Geometry: see drawing. Coordinates: mm, zero at the bounding-box minimum. A direction names the side the tool comes from. Give positions to 0.01 mm unless a question says otherwise; leave off trailing zeros. Loops run counter-clockwise (first coordinate to the right, second up) from the corner with the lowest first, then second, coordinate; pieces in that order, holes last. Notation, with made-up numbers: M 18.5,-17 L 55.5,-17 A14 ccw 55.5,2 Z; hole C 22.5,-9.5 d1. An arc over 180 degrees is marked long. Put each result on its own line as item: value.
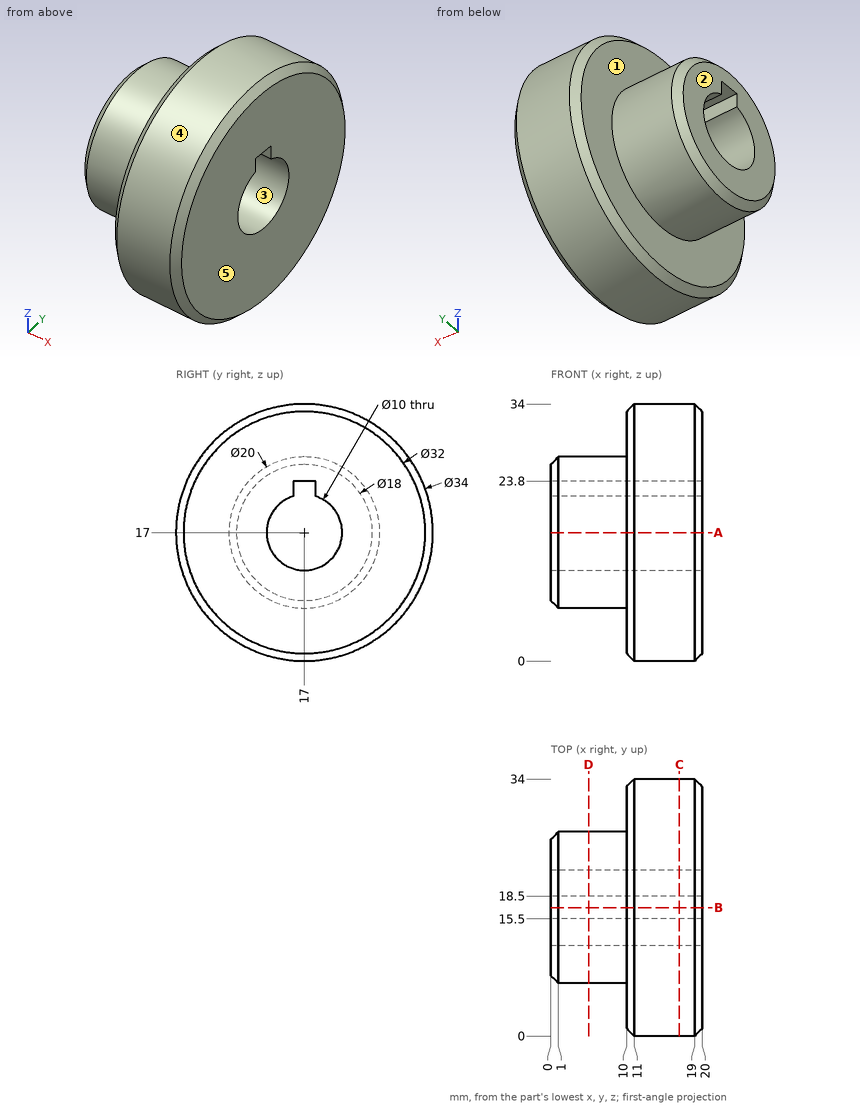
1. Material intervals for line 1 (Y direction, x = 16, z = 17); line 2 (Z direction, x = 4.75, y = 17); line 3 (Z direction, x = 12.5, y = 17), sorted ascending. Write a range as from..to.
Found:
line 1: 0..12, 22..34
line 2: 7..12, 23.8..27
line 3: 0..12, 23.8..34
2. Section query B-B (y = 17). Output: boundary loops of the cut face in (x, z).
Found:
outline: M 0,8 L 1,7 L 10,7 L 10,1 L 11,0 L 19,0 L 20,1 L 20,12 L 0,12 Z; M 0,23.8 L 20,23.8 L 20,33 L 19,34 L 11,34 L 10,33 L 10,27 L 1,27 L 0,26 Z
3. Access query for the marked faces 1 and 2. Directions: +Z, -Z, +X, -X, +Y, -Y. A direction counts if a zero-diameter tool reaches every point of the face in a straight line with its end or side. Return the directions, or none.
Found:
face 1: -X
face 2: +Z, -Z, -X, +Y, -Y
4. Section query D-D (x = 5). Output: boundary loops of the cut face in (y, z), plus the area to 3 significant figures.
Found:
outline: C 17,17 d20; hole M 15.5,21.77 A5 ccw long 18.5,21.77 L 18.5,23.8 L 15.5,23.8 Z
area: 230 mm^2
5. Section query C-C (x = 17). Output: boundary loops of the cut face in (y, z), plus the area to 3 significant figures.
Found:
outline: C 17,17 d34; hole M 15.5,21.77 A5 ccw long 18.5,21.77 L 18.5,23.8 L 15.5,23.8 Z
area: 824 mm^2
6. Section query A-A (z = 17). Output: boundary loops of the cut face in (x, y), plus the area to 3 significant figures.
Found:
outline: M 0,8 L 1,7 L 10,7 L 10,1 L 11,0 L 19,0 L 20,1 L 20,12 L 0,12 Z; M 0,22 L 20,22 L 20,33 L 19,34 L 11,34 L 10,33 L 10,27 L 1,27 L 0,26 Z
area: 337 mm^2
7. Draft query along Z for the marked faces 3, 4 and 5. Return one class per face: pulls with the +Z half, pulls with the -Z half, needs draft (parallel to the pull), parting line crosses it, or undercut.
Found:
face 3: undercut
face 4: parting line crosses it
face 5: needs draft
8. Contact query for flat-ended pins moving along their axis: P1, Ø6, axis at y = 17, z = 17, coming from the +X side; P2, Ø8, axis at x = 11.5, z = 16, coming from the +Y side; P3, Ø1, axis at x = 5, z = 23, coming from the +Y side; P4, Ø0.9, axis at x = 8.5, y = 16.5, coming from the -Z side. Output: stop coordinate, or through.
Found:
P1: through
P2: y = 34
P3: y = 25.35
P4: z = 7
